Autodesk Inventor part; units mm, degrees
ref_plane "YZ Plane" through (0, 0, 0) normal (1, 0, 0) x (0, 1, 0)
ref_plane "XZ Plane" through (0, 0, 0) normal (0, 1, 0) x (-1, 0, 0)
ref_plane "XY Plane" through (0, 0, 0) normal (0, 0, 1) x (1, 0, 0)
sketch "Sketch1" plane through (0, 0, 0) normal (0, 1, 0) x (-1, 0, 0)
  line L0 (10, 0.3) -> (-10, 0.3)
  line L1 (-10, 0.3) -> (-10, 0)
  line L2 (-10, 0) -> (10, 0)
  line L3 (10, 0) -> (10, 0.3)
  line L4 (-6.5, 0.3) -> (6.5, 0.3)
  line L5 (6.5, 0.3) -> (6.5, 8.7)
  line L6 (6.5, 8.7) -> (-6.5, 8.7)
  line L7 (-6.5, 8.7) -> (-6.5, 0.3)
  line L8 (6.5, 8.7) -> (5, 8.7)
  line L9 (0.4, 8.7) -> (0.4, 13.5)
  line L10 (-0.4, 13.5) -> (-0.4, 8.7)
  line L11 (-4.2, 13.5) -> (-4.2, 8.7)
  line L12 (-5, 8.7) -> (-5, 13.5)
  line L13 (4.2, 13.5) -> (4.2, 8.7)
  line L14 (5, 8.7) -> (5, 13.5)
  line L15 (4.2, 13.5) -> (5, 13.5)
  line L16 (-5, 13.5) -> (-4.2, 13.5)
  line L17 (-0.4, 13.5) -> (0.4, 13.5)
  line L18 (4.2, 8.7) -> (-6.5, 8.7)
  line L19 (5, 8.7) -> (4.2, 8.7)
  point P0 (0, 0)
  point P1 (0, 0)
  dimension "d0" = 20
  dimension "d1" = 0.3
  dimension "d2" = 13
  dimension "d6" = 8.7
  dimension "d7" = 13.5
extrude "Extrusion1" add sketch "Sketch1" along normal mid plane 7 contours L0 L7 L6 L5
extrude "Extrusion2" add sketch "Sketch1" along normal mid plane 6.1 contours L3 L2 L1 L0
extrude "Extrusion3" add sketch "Sketch1" along normal mid plane 2 contours L6 L13 L15 L14 | L12 L16 L11 L6 | L6 L10 L17 L9
sketch "Sketch2" plane through (10, 3.05, 0) normal (0, 0, -1) x (-1, 0, 0)
  line L0 (0, -6.1) -> (0, 0)
  line L1 (20, -6.1) -> (20, 0)
  line L2 (20, -6.1) -> (0, -6.1)
  line L3 (0, 0) -> (20, 0)
  arc A0 (18.75, -1.8) -> (18.75, -4.3) centre (18.75, -3.05) ccw
  line L4 (18.75, -4.3) -> (20, -4.3)
  line L5 (18.75, -1.8) -> (20, -1.8)
  arc A1 (1.25, -4.3) -> (1.25, -1.8) centre (1.25, -3.05) ccw
  line L6 (1.25, -4.3) -> (0, -4.3)
  line L7 (1.25, -1.8) -> (0, -1.8)
  line L8 (13.05, -1.1) -> (6.95, -1.1)
  line L9 (6.95, -1.1) -> (6.95, -5)
  line L10 (6.95, -5) -> (13.05, -5)
  line L11 (13.05, -5) -> (13.05, -1.1)
  line L12 (13.05, -1.1) -> (9.25, -1.1)
  line L13 (9.25, -1.1) -> (9.25, -5)
  line L14 (9.25, -5) -> (13.05, -5)
  line L15 (13.05, -5) -> (13.05, -1.1)
  line L16 (0, -1.8) -> (0, -4.3)
  line L17 (20, -1.8) -> (20, -4.3)
  line L18 (3.5, 0.45) -> (16.5, 0.45)
  line L19 (16.5, -6.55) -> (3.5, -6.55)
  point P0 (10, -3.05)
  dimension "d16" = 6.1
  dimension "d17" = 2.5
  dimension "d18" = 17.5
  dimension "d22" = 3.9
  dimension "d23" = 6.1
  dimension "d24" = 3.8
  dimension "d34" = 7
extrude "Extrusion4" cut sketch "Sketch2" against normal blind 0.3 contours L0 L7 A1 L6 | L4 A0 L5 L1
extrude "Extrusion5" add sketch "Sketch2" along normal blind 5 contours L11 L10 L13 L8
fillet "Fillet1" radius 0.5 2 edges at (0.75, 0, -5) (-3.05, 0, -5)
sketch "Sketch3" plane through (-5, -1, 13.5) normal (-1, 0, 0) x (0, 0, 1)
  line L0 (-0.5, 0.5) -> (-2.3, 0.5)
  line L1 (-2.3, 0.5) -> (-2.3, 1.5)
  line L2 (-2.3, 1.5) -> (-0.5, 1.5)
  line L3 (-0.5, 1.5) -> (-0.5, 0.5)
  point P0 (-13.5, 1)
  dimension "d30" = 1.8
  dimension "d31" = 1
extrude "Extrusion6" cut sketch "Sketch3" against normal blind 13
properties part number "Power_Switch"
CAD build for the part. Positions are in the model's coordinates, mm. A direction names the side the tool comes from. Give positions to 0.01 mm unless a question says otherwise; leave off trailing zeros. Write each loop counter-clockwise with the first axis right and the second up, starting at its lowest first coordinate (ties: lowest second). Pieces come first, ordered by that corner, then holes. Notation, with made-up numbers: (23, 39.5) -> (52, 39.5) arc R14 cw to (52, 54.5) -> close; hole circle Ø6 at (62, 26.25). An arc over 180 degrees is marked (long way). Write each question's results on one line, items separated by ' | '.
1. Cut at D-D, the plane x = 6.25. Write the cut outline in (y, z).
Geometry check:
outline: (-3.5, 0.3) -> (-3.05, 0.3) -> (-3.05, 0) -> (3.05, 0) -> (3.05, 0.3) -> (3.5, 0.3) -> (3.5, 8.7) -> (-3.5, 8.7) -> close
2. Wall check: probe 1 along X at (y, z) = (-1.5, 1.75); probe 2 along Z at (x, y) = (4.25, 3); probe 3 along X at (y, z) = (1, -2.75). Give the ranges that are in metal, low to high. Write a range as [from, to].
Geometry check:
probe 1: [-6.5, 6.5] | probe 2: [0, 8.7] | probe 3: [-3.05, 0.75]
3. Drop flat-ended pins along their axis: P1, Ø1.5, axis at y = 0.5, z = 9, coming from the -X side; P2, Ø4, axis at x = -1, z = -3.5, coming from the -Y side; P3, Ø0.9, axis at x = 4.5, z = 12, coming from the +Y side. Give the stop position or say it passes through.
Geometry check:
P1: x = -6.5 | P2: y = -1.95 | P3: y = 1
4. Which spindle directions (+Z, -Z, +X, -X, +Y, -Y) get a long thin tool onto all of the face, cutting with end or side? Do faces 4 (the flat face through (0, 0, 11.2)), 5 (the flat face through (-5, 0, 11)), 6 (the flat face through (-4.2, 0, 11)). Say none if no direction does.
Geometry check:
face 4: +X, -X | face 5: +Z, -X, +Y, -Y | face 6: +Z, +Y, -Y
5. Cut at A-A, the plane x = 9. Write the cut outline in (y, z), then the cut area to 3 significant figures.
Geometry check:
outline: (-3.05, 0) -> (-1.25, 0) -> (-1.25, 0.3) -> (-3.05, 0.3) -> close; (1.25, 0) -> (3.05, 0) -> (3.05, 0.3) -> (1.25, 0.3) -> close | area: 1.08 mm²
6. Cut at C-C, the plane z = 11.5. Write the cut outline in (x, y).
Geometry check:
outline: (-5, -1) -> (-4.2, -1) -> (-4.2, -0.5) -> (-5, -0.5) -> close; (-5, 0.5) -> (-4.2, 0.5) -> (-4.2, 1) -> (-5, 1) -> close; (-0.4, -1) -> (0.4, -1) -> (0.4, -0.5) -> (-0.4, -0.5) -> close; (-0.4, 0.5) -> (0.4, 0.5) -> (0.4, 1) -> (-0.4, 1) -> close; (4.2, -1) -> (5, -1) -> (5, -0.5) -> (4.2, -0.5) -> close; (4.2, 0.5) -> (5, 0.5) -> (5, 1) -> (4.2, 1) -> close
7. Cut at B-B, the plane z = 9. Write the cut outline in (x, y), then the cut area to 3 significant figures.
Geometry check:
outline: (-5, -1) -> (-4.2, -1) -> (-4.2, 1) -> (-5, 1) -> close; (-0.4, -1) -> (0.4, -1) -> (0.4, 1) -> (-0.4, 1) -> close; (4.2, -1) -> (5, -1) -> (5, 1) -> (4.2, 1) -> close | area: 4.80 mm²
8. Two-plate mould, pull along Y, no slides. Class faces 1 (the flat face through (4.6, 1, 11.1)), 2 (the flat face through (4.6, 0, 13)), 3 (the flat face through (-0.4, 0, 11)): pulls with the +Y half, pulls with the -Y half, needs draft (parallel to the pull), parting line crosses it, or undercut.
Geometry check:
face 1: pulls with the +Y half | face 2: undercut | face 3: needs draft
